Verification items for this drawing (mm, ordinates from the low corner). A direction names the side the tool comes from. Round coordinates to 2 decimals unless told otherwise and drop trailing zeros. Order: outer loops, then holes, each group sorted by start corner. A loop starts at its lowest first (then second) coordinate and runs counter-clockwise, first axis right, second up.
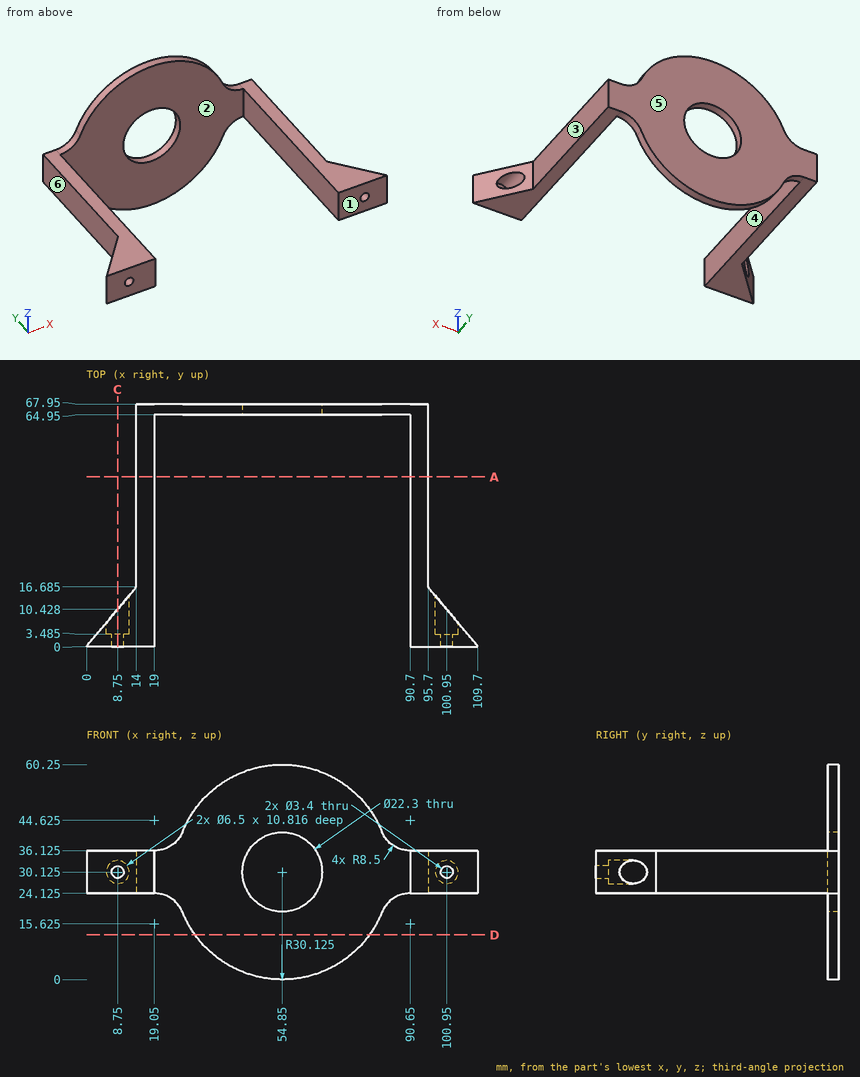
Item 1: Sectioned sample at C-C (x = 8.75). Record the cut outline in (y, z) (1 decimal).
Answer:
outline: (0, 24.1) - (10.4, 24.1) - (10.4, 26.9) - (3.5, 26.9) - (3.5, 28.4) - (0, 28.4) - close; (0, 31.8) - (3.5, 31.8) - (3.5, 33.4) - (10.4, 33.4) - (10.4, 36.1) - (0, 36.1) - close
Item 2: Release check for a two-part mould opening along X. For the marked faces 3, 4, 5 and 6 record: released by +X, released by -X, zero draft, split by the parting line, or undercut.
Answer:
face 3: released by +X
face 4: undercut
face 5: zero draft
face 6: released by -X
Item 3: Go/stop test with flat-tipped pins: P1, Ø2, axis at x = 99.5, z = 30.5, coming from the +Y side (1 decimal); P2, Ø10, axis at y = 57, z = 40.5, coming from the -X side; P3, Ø2.5, axis at x = 100.95, z = 30.125, coming from the -Y side; P4, Ø12, axis at x = 25.5, z = 41.5, coming from the -Y side. Record where each tip stops, or that it passes through.
Answer:
P1: stops at y = 3.5
P2: stops at x = 14
P3: passes through
P4: stops at y = 64.95
Item 4: Scan lines: line 1 along Z through (x, y) = (100.95, 2.2) (1 decimal); line 2 along X through (y, z) = (55, 29.5); line 3 along Z through (x, y) = (100.95, 10.25) (1 decimal). Record each from-to range of solid material in increasing order.
Answer:
line 1: z = 24.1 to 28.4, 31.8 to 36.1
line 2: x = 14 to 19, 90.7 to 95.7
line 3: z = 24.1 to 26.9, 33.4 to 36.1
Item 5: Sectioned sample at A-A (y = 47.5). Record the cut outline in (x, z) (1 decimal), and give its area (3 significant figures).
Answer:
outline: (14, 24.1) - (19, 24.1) - (19, 36.1) - (14, 36.1) - close; (90.7, 24.1) - (95.7, 24.1) - (95.7, 36.1) - (90.7, 36.1) - close
area: 120 mm2
Item 6: Sectioned sample at D-D (z = 12.5). Record the cut outline in (x, y).
Answer:
outline: (30.42, 64.95) - (79.28, 64.95) - (79.28, 67.95) - (30.42, 67.95) - close
Item 7: Access from +Z, -Z, +X, -X, +Y, -Y to the whole of each face (thin tool, end or side, straight path). Record for the marked faces 1 and 2.
Answer:
face 1: +Z, -Z, +X, -X, -Y
face 2: +Z, -Z, -Y
